```python
from build123d import *

# Parameters (mm, degrees)
SKETCH_5_W          = 20
SKETCH_5_H          = 30
SKETCH_5_R          = 2.75
EXTRUDE_1_DEPTH     = 5
SKETCH_6_W          = 20
SKETCH_6_H          = 5
EXTRUDE_2_DEPTH     = 30
SKETCH_7_R          = 1.8
CUT_EXTRUDE_1_DEPTH = 6


with BuildPart() as part:
    # 草图5 → 凸台-拉伸1 (new body)
    with BuildSketch(Plane(origin=(0, 0, 0), x_dir=(0, 0, -1), z_dir=(1, 0, 0))):
        Rectangle(SKETCH_5_W, SKETCH_5_H)
        with Locations((0, 10)):
            Circle(SKETCH_5_R, mode=Mode.SUBTRACT)
    extrude(amount=EXTRUDE_1_DEPTH)

    # 草图6 → 凸台-拉伸2 (add)
    with BuildSketch(Plane(origin=(5, 0, 0), x_dir=(0, 0, -1), z_dir=(1, 0, 0))):
        with Locations((0, -12.5)):
            Rectangle(SKETCH_6_W, SKETCH_6_H)
    extrude(amount=EXTRUDE_2_DEPTH)

    # 草图7 → 切除-拉伸1 (cut, through all)
    with BuildSketch(Plane(origin=(0, -10, 0), x_dir=(1, 0, 0), z_dir=(0, 1, 0))):
        with Locations((20, 0)):
            Circle(SKETCH_7_R)
    extrude(amount=-CUT_EXTRUDE_1_DEPTH, mode=Mode.SUBTRACT)


solid = part.part
```
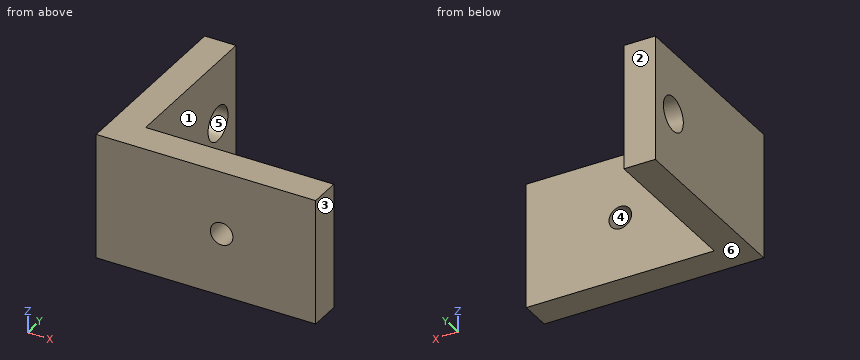
Input: part model. Units: mm. Frame: model coordinates. Face numbers are marked on the shaded views. A direction names the side the tool comes from. Give positions to 0.01 mm unless a question says otherwise; leave off trailing zeros. Order: outer loops, then holes, each group sorted by start corner. A loop starts at its lowest first (then second) coordinate and runs counter-clockwise, first axis right, second up.
1. Cut plane D-D (z = 8.75). Return loops of the section in (x, y), and give its area (3 significant figures).
Computed:
outline: (0, -15) - (35, -15) - (35, -10) - (5, -10) - (5, 15) - (0, 15) - close
area: 300 mm2
2. Cut plane B-B (z = 0). Return loops of the section in (x, y).
Computed:
outline: (0, -15) - (18.2, -15) - (18.2, -10) - (5, -10) - (5, 7.25) - (0, 7.25) - close; (0, 12.75) - (5, 12.75) - (5, 15) - (0, 15) - close; (21.8, -15) - (35, -15) - (35, -10) - (21.8, -10) - close
3. Draft query along Z for the marked faces 3, 4, 5 and 6. Return one class per face: released by +Z, released by -Z, zero draft, split by the parting line, or undercut.
Computed:
face 3: zero draft
face 4: undercut
face 5: undercut
face 6: released by -Z
4. Line query: probe 1 along Y at (x, z) = (3.6, 0); probe 2 along X at (y, z) = (-13.9, 0); probe 3 along X at (y, z) = (4.75, -1.25). Output: solid intervals per line, ascending.
Computed:
probe 1: y = -15 to 7.25, 12.75 to 15
probe 2: x = 0 to 18.2, 21.8 to 35
probe 3: x = 0 to 5
5. Pin query (flat end, axial travel): pin 1 Ø12 at (x, z) = (12.5, -6) entering from +Y; pin 2 Ø10 at (y, z) = (6, 5) entering from +X. Return the tip coordinate at first contact, or that it passes through.
Computed:
pin 1: stops at y = -10
pin 2: stops at x = 5
6. Set-up query: the marked faces 1 and 2. Return all of +Z, -Z, +X, -X, +Y, -Y with unobstructed straight access to the full face (end or side cutting, diameter ignored); none if empty.
Computed:
face 1: +Z, -Z, +X, +Y
face 2: +Z, -Z, +X, -X, +Y
7. Cut plane A-A (y = 10). Return loops of the section in (x, z).
Computed:
outline: (0, -10) - (5, -10) - (5, -2.75) - (0, -2.75) - close; (0, 2.75) - (5, 2.75) - (5, 10) - (0, 10) - close
8. Cut plane C-C (x = 20). Return loops of the section in (y, z), and give its area (3 significant figures).
Computed:
outline: (-15, -10) - (-10, -10) - (-10, -1.8) - (-15, -1.8) - close; (-15, 1.8) - (-10, 1.8) - (-10, 10) - (-15, 10) - close
area: 82.0 mm2
